```python
from build123d import *

# Parameters (mm, degrees)
SKETCH1_R               = 13
SKETCH1_R_2             = 5
SKETCH1_W               = 10
SKETCH1_H               = 100
SKETCH1_W_2             = 15
SKETCH1_H_2             = 15
BOSS_EXTRUDE1_DEPTH     = 4.5
SKETCH2_R               = 11
CUT_EXTRUDE1_DEPTH      = 7
FILLET7_R               = 1
FILLET1_R               = 20
CUT_EXTRUDE2_DEPTH      = 113.841703284
CUT_EXTRUDE2_DEPTH_BACK = 113.841703284
SKETCH3_W               = 4.5
SKETCH3_H               = 90.459340771
M3_CLEARANCE_HOLE1_D    = 3.4
FILLET5_R               = 4.5
FILLET6_R               = 4.5
BOSS_EXTRUDE2_DEPTH     = 2
FILLET8_R               = 1
FILLET9_R               = 1


# Some blends are built 0.0001 mm under size
with BuildPart() as part:
    # Sketch1 → Boss-Extrude1 (new, symmetric)
    # profile 1 of 3: a face of its own
    with BuildSketch(Plane.XY):
        Circle(SKETCH1_R)
        Circle(SKETCH1_R_2, mode=Mode.SUBTRACT)
    # profile 2 of 3: a face of its own
    with BuildSketch(Plane.XY):
        with Locations((0, 62)):
            Rectangle(SKETCH1_W, SKETCH1_H)
    # profile 3 of 3: a face of its own
    with BuildSketch(Plane.XY):
        with Locations((0, 104.5)):
            Rectangle(SKETCH1_W_2, SKETCH1_H_2)
    extrude(amount=BOSS_EXTRUDE1_DEPTH, both=True)

    # Sketch2 → Cut-Extrude1 (cut)
    with BuildSketch(Plane(origin=(0, 0, -4.5), x_dir=(-1, 0, 0), z_dir=(0, 0, -1))):
        Circle(SKETCH2_R)
    extrude(amount=-CUT_EXTRUDE1_DEPTH, mode=Mode.SUBTRACT)

    # Fillet7
    fillet7_edges = [part.edges().sort_by_distance(p)[0] for p in [
        (-5, 97, 0),
        (5, 97, 0),
        (7.5, 97, 0),
        (7.5, 112, 0),
        (-7.5, 112, 0),
        (-7.5, 97, 0),
    ]]
    fillet(fillet7_edges, radius=FILLET7_R)

    # Fillet1
    fillet1_edges = [part.edges().sort_by_distance(p)[0] for p in [
        (-5, 12, 0),
        (5, 12, 0),
    ]]
    fillet(fillet1_edges, radius=FILLET1_R)

    # Sketch3 → Cut-Extrude2 (cut, two sides: drawn at the far end of the back side and taken through both)
    with BuildSketch(Plane(origin=(0, 0, 0), x_dir=(0, 0, -1), z_dir=(1, 0, 0)).offset(-CUT_EXTRUDE2_DEPTH_BACK)):
        with Locations((2.25, 66.770329614)):
            Rectangle(SKETCH3_W, SKETCH3_H)
    extrude(amount=CUT_EXTRUDE2_DEPTH + CUT_EXTRUDE2_DEPTH_BACK, mode=Mode.SUBTRACT)

    # M3 Clearance Hole1 (through all)
    with Locations(Plane.XY.offset(4.5)):
        with Locations((3, 99), (-3, 105)):
            Hole(M3_CLEARANCE_HOLE1_D / 2)

    # Fillet5
    fillet5_edges = [part.edges().sort_by_distance(p)[0] for p in [
        (0, 21.540659229, 0),
    ]]
    fillet(fillet5_edges, radius=FILLET5_R - 0.0001)  # a hair under: the kernel refuses the full size

    # Fillet6
    # the kernel refuses this fillet: 4.5 mm, written as the material it takes off along each edge
    with BuildSketch(Plane(origin=(-13.235677247, 21.540659229, -4.5), x_dir=(0, -1, 0), z_dir=(1, 0, 0))) as fillet6_piece_1:
        with BuildLine():
            CenterArc((3.294270899, -4.5), FILLET6_R, 90, 60.000367556)
            Line((-0.602857852, -2.250025), (-0.992570727, -2.0250275))
            ThreePointArc((-0.992570727, -2.0250275), (-0.45, -0.0001), (-0.45, 0))
            Line((-0.45, 0), (0, 0.45))
            Line((0, 0.45), (3.294270899, 0.45))
            Line((3.294270899, 0.45), (3.294270899, 0))
        make_face()
    extrude(amount=26.471354494, mode=Mode.SUBTRACT)

    # Sketch10 → Boss-Extrude2 (add)
    with BuildSketch(Plane(origin=(0, 52, 0), x_dir=(-1, 0, 0), z_dir=(0, -1, 0))):
        Polygon((5, -4.5), (7.5, -4.5), (7.5, 6.5), (-7.5, 6.5), (-7.5, -4.5), (-5, -4.5), (-5, 4), (5, 4), align=None)
    extrude(amount=-BOSS_EXTRUDE2_DEPTH)

    # Fillet8
    fillet8_edges = [part.edges().sort_by_distance(p)[0] for p in [
        (-5, 52, -2),
        (5, 54, -2),
        (5, 53, -4),
        (7.5, 52, -1),
        (0, 54, -6.5),
        (7.5, 53, -6.5),
        (-7.5, 54, -1),
        (-7.5, 53, -6.5),
        (0, 52, -4),
        (-5, 53, -4),
        (7.5, 54, -1),
        (-5, 54, -2),
        (0, 54, -4),
        (5, 52, -2),
        (-7.5, 52, -1),
        (0, 52, -6.5),
    ]]
    fillet(fillet8_edges, radius=FILLET8_R - 0.0001)  # a hair under: the kernel refuses the full size

    # Fillet9
    fillet9_edges = [part.edges().sort_by_distance(p)[0] for p in [
        (5, 54, 2.25),
        (-5, 54, 2.25),
        (-5, 52, 2.25),
        (5, 52, 2.25),
    ]]
    fillet(fillet9_edges, radius=FILLET9_R - 0.0001)  # a hair under: the kernel refuses the full size


solid = part.part
```
Here's how the part is built. I have some questions about the finished solid (model axes, mm). A direction names the side the tool comes from. Give positions to 0.01 mm unless a question says otherwise; leave off trailing zeros. Order: outer loops, then holes, each group sorted by start corner. A loop starts at its lowest first (then second) coordinate and runs counter-clockwise, first axis right, second up. Notation, with made-up numbers: (88, -16.5) -> (140, -16.5) arc R17 cw to (140, -6.5) -> close; hole circle Ø5 at (-17.5, 44.25). An arc over 180 degrees is marked (long way). Use CSV: the item, a comma, the result in double quotes. Start each with the question number.
Item 1: Suppose I cut it at B-B (y = 0). List the corners of the cut face in (x, z) for me, and give its area (3 significant figures).
Item 2: On a 3-axis mill with a long thin cutter (end or side, diameter ignored), from which of +Z, -Z, +X, -X, +Y, -Y can I reach the whole of each face in a straight line? I mean faces 1 (the flat face through (-1, 12, -4.5)), 2 (the flat face through (-5, 36, 2)), 3 (the flat face through (0, 54, -5.3)), 4 (the flat face through (5, 36, 2)). Say none if no direction works.
Item 3: Suppose I cut it at D-D (y = 87). List the corners of the cut face in (x, z) for me, and give its area (3 significant figures).
Item 4: Suppose I cut it at C-C (x = -2.5). Give the number of separate pieces and of enclosed holes in the cut face, and give its area (3 significant figures).
Item 5: If I drill on probe 1 along Y at (x, z) = (0, 0.25); probe 2 along Y at (x, z) = (3, 3.4); probe 3 along Y at (x, z) = (-3.25, 1.25), over which ranges is the centre line in solid material (lowest first)? Write a range as [from, to].
Item 6: I'm going to push flat-ended pins straight in: P1, Ø5, axis at x = -5.5, z = -3, coming from the -Y side; P2, Ø6, axis at y = 37.5, z = 2.5, coming from the +X side; P3, Ø1, axis at x = -5, y = 69, coming from the -Z side. Where does each tip first touch, or does it pass through?
Item 7: Thinking about a two-plate mould opening in X: for faces 5 (the cylindrical face through (3.37, 97.34, 2.22)), 6 (the cylindrical face through (6.286, 14.484, 0.063)), 7 (the flat face through (0, 52, -5.3)), which applies, pulls with the +X half, pulls with the -X half, needs draft (parallel to the pull), parting line crosses it, or undercut?
Item 8: Suppose I cut it at A-A (y = 105). List the corners of the cut face in (x, z) for me, and give its area (3 significant figures).
Answer block:
1,outline,"(-13, -4.5) -> (-11, -4.5) -> (-11, 2.5) -> (-5, 2.5) -> (-5, 4.5) -> (-13, 4.5) -> close; (5, 2.5) -> (11, 2.5) -> (11, -4.5) -> (13, -4.5) -> (13, 4.5) -> (5, 4.5) -> close"
1,area,"60.0 mm^2"
2,face 1,"-Z, +X, -X, -Y"
2,face 2,"+Z, -Z, -X"
2,face 3,"-Z"
2,face 4,"+Z, -Z, +X"
3,outline,"(-5, 0) -> (5, 0) -> (5, 4.5) -> (-5, 4.5) -> close"
3,area,"45.0 mm^2"
4,separate pieces,"4"
4,enclosed holes,"0"
4,area,"541 mm^2"
5,probe 1,"y = [-13, -11], [11, 112]"
5,probe 2,"y = [-12.65, -4], [4, 97.3], [100.7, 112]"
5,probe 3,"y = [-12.59, -10.51], [10.51, 103.32], [106.68, 112]"
6,P1,"stops at y = -12.65"
6,P2,"stops at x = 5"
6,P3,"stops at z = 0"
7,face 5,"undercut"
7,face 6,"pulls with the +X half"
7,face 7,"needs draft"
8,outline,"(-7.5, 0) -> (-4.7, 0) -> (-4.7, 4.5) -> (-7.5, 4.5) -> close; (-1.3, 0) -> (7.5, 0) -> (7.5, 4.5) -> (-1.3, 4.5) -> close"
8,area,"52.2 mm^2"
